```python
from build123d import *

# Parameters (mm, degrees)
F0_R       = 14.5692591233
F0_R_2     = 9.7754481422
F1_DEPTH   = 25
F2_DEPTH   = 50
F3_C1_SIZE = 2
F3_C2_SIZE = 2
F3_C3_SIZE = 1.9999
F3_C4_SIZE = 1.9999
F3_C5_SIZE = 1.9999
F4_SIZE    = 5


# Not quite as in the source:
# - a fillet or chamfer is up to 0.001 mm smaller than in the source, because OpenCascade refuses the exact size


with BuildPart() as f1:
    # F0 (on Front) → F1 (new body)
    with BuildSketch(Plane.XZ):
        with BuildLine():
            Line((5.4392563459, 24.4011165811), (0, 25))
            ThreePointArc((0, 25), (-25, 0), (0, -25))
            Line((0, -25), (5.487804878, -24.3902439024))
            ThreePointArc((5.487804878, -24.3902439024), (19.5217202361, -15.6173761889), (25, 0))
            ThreePointArc((25, 0), (19.5061709293, 15.6367930113), (5.4392563459, 24.4011165811))
        make_face()
        Circle(F0_R, mode=Mode.SUBTRACT)
        with BuildLine():
            ThreePointArc((5.4392563459, 24.4011165811), (2.7360633648, 24.8498281134), (0, 25))
            Line((0, 25), (5.4392563459, 24.4011165811))
        make_face()
        with BuildLine():
            Line((5.487804878, -24.3902439024), (0, -25))
            ThreePointArc((0, -25), (2.7607881519, -24.8470933668), (5.487804878, -24.3902439024))
        make_face()
        with BuildLine():
            Line((91.6416380189, 14.909896868), (5.4392563459, 24.4011165811))
            ThreePointArc((5.4392563459, 24.4011165811), (19.5061709293, 15.6367930113), (25, 0))
            ThreePointArc((25, 0), (19.5217202361, -15.6173761889), (5.487804878, -24.3902439024))
            Line((5.487804878, -24.3902439024), (90, -15))
            ThreePointArc((90, -15), (75.0225427221, 0.8220544324), (91.6416380189, 14.909896868))
        make_face()
        with BuildLine():
            ThreePointArc((105, 0), (101.1719418698, 10.0093813424), (91.6416380189, 14.909896868))
            ThreePointArc((91.6416380189, 14.909896868), (75.0225427221, 0.8220544324), (90, -15))
            ThreePointArc((90, -15), (100.6066017178, -10.6066017178), (105, 0))
        make_face()
        with Locations((90, 0)):
            Circle(F0_R_2, mode=Mode.SUBTRACT)
    extrude(amount=F1_DEPTH)

    # F0 (on Front) → F2 (join)
    with BuildSketch(Plane.XZ):
        with BuildLine():
            Line((5.4392563459, 24.4011165811), (0, 25))
            ThreePointArc((0, 25), (-25, 0), (0, -25))
            Line((0, -25), (5.487804878, -24.3902439024))
            ThreePointArc((5.487804878, -24.3902439024), (19.5217202361, -15.6173761889), (25, 0))
            ThreePointArc((25, 0), (19.5061709293, 15.6367930113), (5.4392563459, 24.4011165811))
        make_face()
        Circle(F0_R, mode=Mode.SUBTRACT)
    extrude(amount=F2_DEPTH)

    # F3: chamfer of 2 on 5 edges, made by hand

    # F3_c1
    f3_c1_edges = [f1.edges().sort_by_distance(p)[0] for p in [
        (-14.5692591233, -50, 0),
    ]]
    chamfer(f3_c1_edges, length=F3_C1_SIZE)

    # F3_c2
    f3_c2_edges = [f1.edges().sort_by_distance(p)[0] for p in [
        (-25, -50, 0),
    ]]
    chamfer(f3_c2_edges, length=F3_C2_SIZE)

    # F3_c3 (size 2 in the source; OpenCascade refuses exactly that, so slightly less here)
    f3_c3_edges = [f1.edges().sort_by_distance(p)[0] for p in [
        (3.7377861737, -50, -24.5846904251),
    ]]
    chamfer(f3_c3_edges, length=F3_C3_SIZE)

    # F3_c4 (size 2 in the source; OpenCascade refuses exactly that, so slightly less here)
    f3_c4_edges = [f1.edges().sort_by_distance(p)[0] for p in [
        (3.7136212975, -50, 24.591115756),
    ]]
    chamfer(f3_c4_edges, length=F3_C4_SIZE)

    # F3_c5 (size 2 in the source; OpenCascade refuses exactly that, so slightly less here)
    f3_c5_edges = [f1.edges().sort_by_distance(p)[0] for p in [
        (24.9999950028, -50, 0.0158069943),
    ]]
    chamfer(f3_c5_edges, length=F3_C5_SIZE)

    # F4
    f4_edges = [f1.edges().sort_by_distance(p)[0] for p in [
        (80.224552, -25, 0),
    ]]
    chamfer(f4_edges, length=F4_SIZE)


solid = f1.part
```
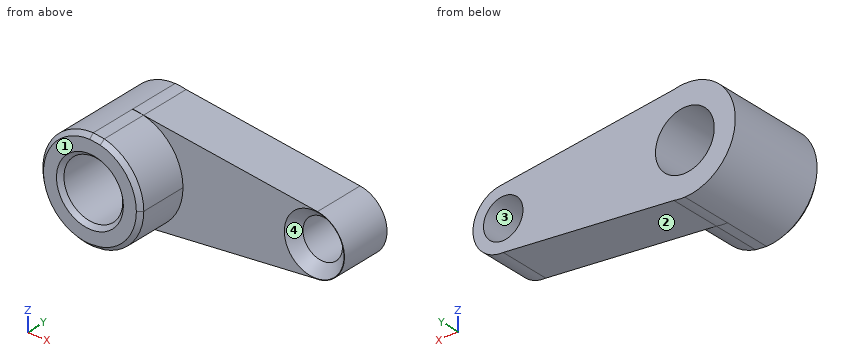
Source: CAD feature listing. Evaluate the final solid. Frame: model axes, mm. Face numbers are marked on the shaded views. Give positions to 0.01 mm unless a question says otherwise; leave off trailing zeros. Order: outer loops, then holes, each group sorted by start corner. A loop starts at its lowest first (then second) coordinate and runs counter-clockwise, first axis right, second up.
(1) Section query A-A (y = -10.5). Return the cut outline in (x, z), plus the area to 3 significant figures.
(2) Section query C-C (z = 8). State how many separate pieces and enclosed holes the cut face has, plus the area to 3 significant figures.
(3) Pull-direction query (X, two-part tool) for the marked faces 1, 2, 3 and 4; classes: +X half, -X half, draft (parallel to the pull), parting line (faces both ways), or undercut.
(4) Section query D-D (x = 27). Return the cut outline in (y, z), plus the area to 3 significant figures.
(5) Material intervals for line 1 along Z through (x, y) = (0, -20); line 2 along X through (y, z) = (-14.5, 9); line 3 along X through (y, z) = (-3, 1), sorted ascending.
(6) Section query B-B (y = -31.5). Return the cut outline in (x, z), plus the area to 3 significant figures.
(7) Contact query for flat-ended pins moving along their axis: P1, Ø0.5, axis at x = 3.5, z = -24.5, coming from the -Y side; P2, Ø4, axis at x = 4, y = -13.5, coming from the +Z side; P3, Ø8, axis at y = -40.5, z = 15.5, coming from the -X side; P4, Ø11.5, axis at x = 90, z = 0, coming from the +Y side. Output: stop coordinate, or through.
Outcome:
1. outline: (5.44, 24.4) arc R25 ccw (long way) to (5.49, -24.39) - (90, -15) arc R15 ccw to (91.64, 14.91) - close; hole circle Ø29.14 at (0, 0); hole circle Ø19.55 at (90, 0)
1. area: 3,970 mm2
2. separate pieces: 3
2. enclosed holes: 0
2. area: 2,800 mm2
3. face 1: draft
3. face 2: +X half
3. face 3: undercut
3. face 4: undercut
4. outline: (-25, -22) - (0, -22) - (0, 22.03) - (-25, 22.03) - close
4. area: 1,100 mm2
5. line 1: z = -25 to -14.57, 14.57 to 25
5. line 2: x = -23.32 to -11.46, 11.46 to 86.18, 93.82 to 102
5. line 3: x = -24.98 to -14.53, 14.53 to 80.28, 99.72 to 104.97
6. outline: (0, -25) - (5.49, -24.39) arc R25 ccw to (5.44, 24.4) - (0, 25) arc R25 ccw to start; hole circle Ø29.14 at (0, 0)
6. area: 1,300 mm2
7. P1: stops at y = -48.36
7. P2: stops at z = 24.92
7. P3: stops at x = -22.2
7. P4: passes through
